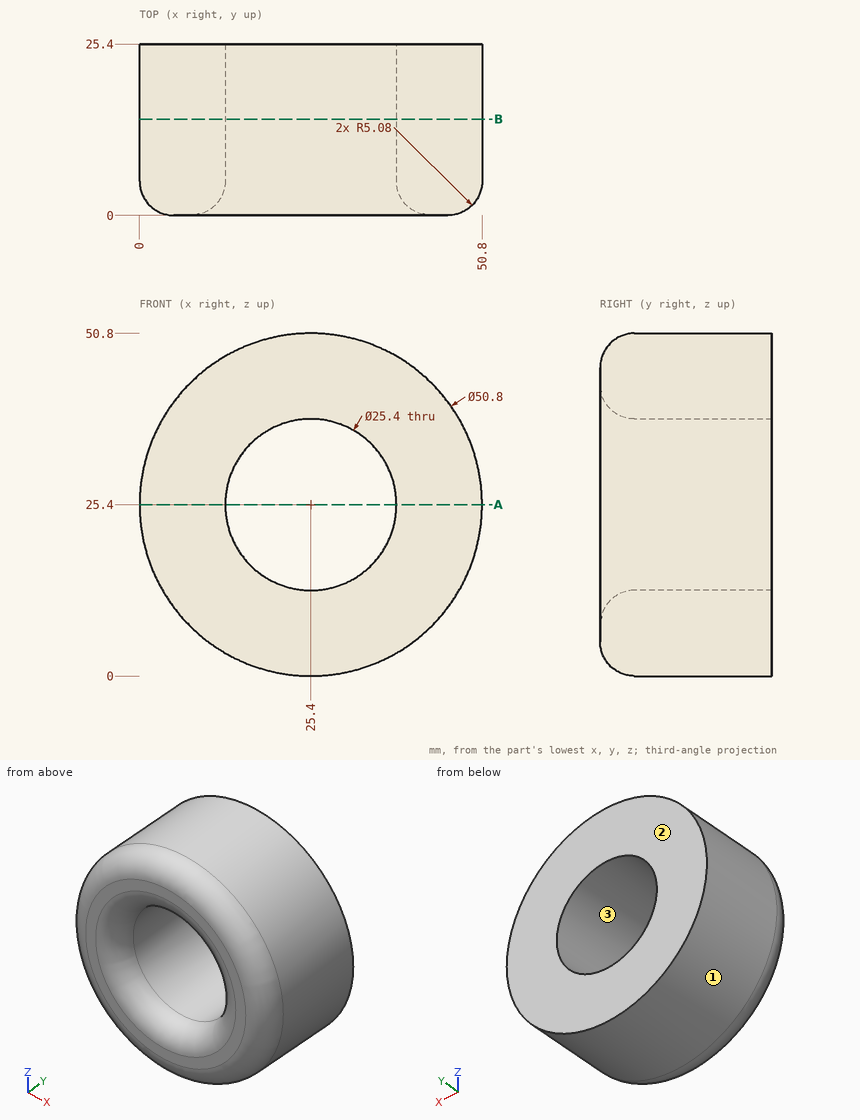
Design review of the part shown in the three views and the two pictorial views. Dimensions are in mm from the part's minimum x, y and z. Coordinates: 2 decimals unless noted, no trailing zeros. Loops run counter-clockwise (first coordinate to the right, second up) from the corner with the lowest first, then second, coordinate; pieces in that order, holes last. Notation, with made-up numbers: M 71,5 L 105,5 A22 ccw 105,17 Z; hole C 52,-37 d9. An arc over 180 degrees is marked long. One line per question, with ' | ' between items.
(1) For pin 1 Ø6 at (y, z) = (9.5, 31.5) entering from +X; pin 2 Ø1 at (x, y) = (28.5, 11) entering from -Z; pin 3 Ø3 at (x, y) = (29, 14) entering from +Z; pin 4 Ø4 at (x, z) = (17, 31.5) entering from -Y, all flat-tipped, find the tip position at first contact; note any pin that passes through.
Filled in:
pin 1: stops at x = 50.61 | pin 2: stops at z = 0.13 | pin 3: stops at z = 50.71 | pin 4: passes through
(2) Draft analysis for pull direction X (two halves, no side actions). For the marked faces 1, 2 and 3, state which applies: released by +X, released by -X, zero draft, split by the parting line, or undercut.
Filled in:
face 1: split by the parting line | face 2: zero draft | face 3: undercut
(3) We need section A-A (z = 25.4). Give the boundary of the cut face in (x, y), and give its area (3 significant figures).
Filled in:
outline: M 0,5.08 A5.08 ccw 5.08,0 L 7.62,0 A5.08 ccw 12.7,5.08 L 12.7,25.4 L 0,25.4 Z; M 38.1,5.08 A5.08 ccw 43.18,0 L 45.72,0 A5.08 ccw 50.8,5.08 L 50.8,25.4 L 38.1,25.4 Z | area: 623 mm^2
(4) We need section B-B (y = 14.25). Give the boundary of the cut face in (x, z), and give its area (3 significant figures).
Filled in:
outline: C 25.4,25.4 d50.8; hole C 25.4,25.4 d25.4 | area: 1,520 mm^2
(5) Wall thickness on probe 1 along Z at (x, y) = (25.4, 15.5); probe 2 along Z at (x, y) = (20.5, 12.25); probe 3 along X at (y, z) = (15, 28): over which ranges is each line inside the solid? List them lowest first.
Filled in:
probe 1: z = 0 to 12.7, 38.1 to 50.8 | probe 2: z = 0.48 to 13.68, 37.12 to 50.32 | probe 3: x = 0.13 to 12.97, 37.83 to 50.67
